Part print with two shaded views. Sizes in mm from the minimum x, y, z corner. Give positions to 0.01 mm unless a question says otherwise; leave off trailing zeros. Write each loop counter-clockwise with the first axis right and the second up, starting at its lowest first coordinate (ties: lowest second). Pieces come first, ordered by that corner, then holes.
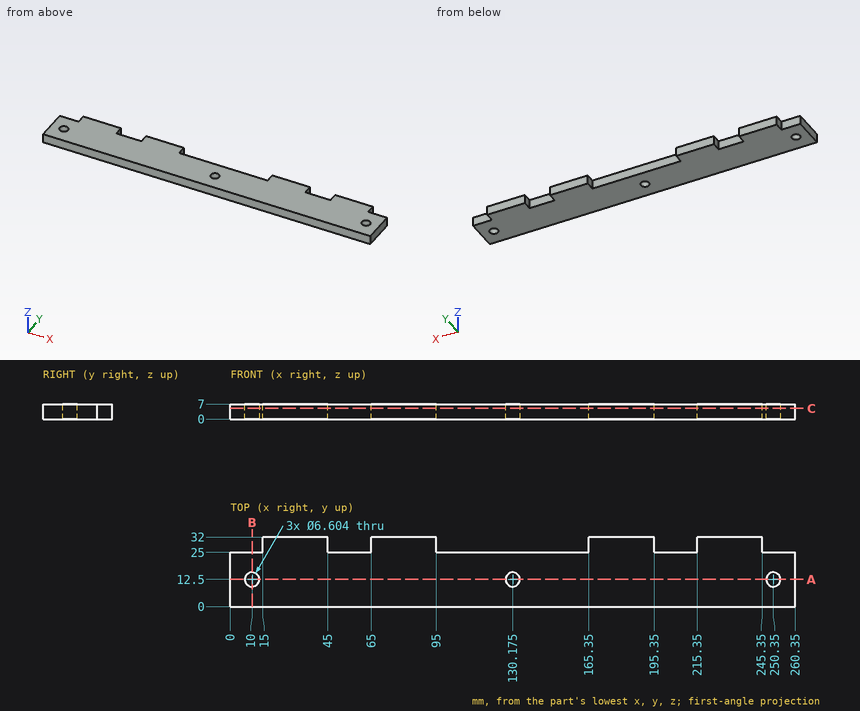
(1) Drop flat-ended pins along their axis: pin 1 (2 mm diameter, centred on y = 28, z = 3, fed in from +X); pin 2 (3.5 mm diameter, centred on x = 202, z = 2, fed in from +Y); pin 3 (3.5 mm diameter, centred on y = 27, z = 5, fed in from -X). Give the stop position or say it passes through.
(2) Saw through at B-B, the plane x = 10. List the corners of the cut face in (y, z), plus the area to 3 significant figures.
(3) Saw through at C-C, the plane z = 5. List the corners of the cut face in (x, y) (3 decimals).
(4) Saw through at A-A, the plane y = 12.5. List the corners of the cut face in (x, z).
(5) Probe line 1 (X direction, y = 28, z = 6); line 2 (X direction, y = 13, z = 2.75); line 3 (Y direction, x = 250.35, z = 5.5). List the from-to ranges inside material, lowest first.
Computed values:
1. pin 1: stops at x = 245.35
1. pin 2: stops at y = 25
1. pin 3: stops at x = 15
2. outline: (0, 0) - (9.2, 0) - (9.2, 7) - (0, 7) - close; (15.8, 0) - (25, 0) - (25, 7) - (15.8, 7) - close
2. area: 129 mm2
3. outline: (0, 0) - (260.35, 0) - (260.35, 25) - (245.35, 25) - (245.35, 32) - (215.35, 32) - (215.35, 25) - (195.35, 25) - (195.35, 32) - (165.35, 32) - (165.35, 25) - (95, 25) - (95, 32) - (65, 32) - (65, 25) - (45, 25) - (45, 32) - (15, 32) - (15, 25) - (0, 25) - close; hole circle Ø6.604 at (10, 12.5); hole circle Ø6.604 at (130.175, 12.5); hole circle Ø6.604 at (250.35, 12.5)
4. outline: (0, 0) - (6.7, 0) - (6.7, 7) - (0, 7) - close; (13.3, 0) - (126.87, 0) - (126.87, 7) - (13.3, 7) - close; (133.48, 0) - (247.05, 0) - (247.05, 7) - (133.48, 7) - close; (253.65, 0) - (260.35, 0) - (260.35, 7) - (253.65, 7) - close
5. line 1: x = 15 to 45, 65 to 95, 165.35 to 195.35, 215.35 to 245.35
5. line 2: x = 0 to 6.74, 13.26 to 126.91, 133.44 to 247.09, 253.61 to 260.35
5. line 3: y = 0 to 9.2, 15.8 to 25
